Design review of the part built by this model. Coordinates are the model's own, in mm. A direction names the side the tool comes from. Give positions to 0.01 mm unless a question says otherwise; leave off trailing zeros. Write each loop counter-clockwise with the first axis right and the second up, starting at its lowest first coordinate (ties: lowest second). Pieces come first, ordered by that corner, then holes. Notation, with made-up numbers: (21.25, -34) -> (38.25, -34) arc R34 ccw to (38.25, 1) -> close; hole circle Ø10 at (55.25, -35). An arc over 180 degrees is marked (long way). Answer as a JSON object with one key per item and string values.
Autodesk Fusion 360 part; units mm, degrees
sketch "Sketch1" plane through (0, 0, 0) normal (0, 0, 1) x (1, 0, 0)
sketch "Sketch2" plane through (0, 0, 0) normal (0, 0, 1) x (1, 0, 0)
  line L0 (0, 0) -> (24, 0)
  line L1 (24, 0) -> (24, 5)
  line L2 (24, 5) -> (0, 5)
  line L3 (0, 5) -> (0, 0)
  dimension "d157" = 24
  dimension "d158" = 5
extrude "Extrude1" add sketch "Sketch2" along normal blind 70
sketch "Sketch3" plane through (0, 0, 0) normal (0, -1, 0) x (1, 0, 0)
  circle A0 centre (12, 8) radius 3
  line L0 (0, 0) -> (24, 0)
  line L1 (0, 0) -> (0, 70)
  dimension "d161" = 6
  dimension "d162" = 8
  dimension "d163" = 12
extrude "Extrude2" cut sketch "Sketch3" against normal blind 5
sketch "Sketch4" plane through (0, 0, 0) normal (0, -1, 0) x (1, 0, 0)
sketch "Sketch5" plane through (0, 0, 0) normal (0, -1, 0) x (1, 0, 0)
  circle A0 centre (12, 8) radius 3
  dimension "d166" = 6
sketch "Sketch6" plane through (0, 0, 70) normal (0, 0, 1) x (-1, 0, 0)
  line L0 (39, -9) -> (-63, -9)
  line L1 (-63, -9) -> (-63, 37)
  line L2 (-63, 37) -> (39, 37)
  line L3 (39, 37) -> (39, -9)
  line L4 (-24, 0) -> (-24, -5)
  line L5 (-24, -5) -> (0, -5)
  line L6 (33, 4) -> (-57, 4)
  line L7 (-57, 4) -> (-57, 24)
  line L8 (-57, 24) -> (33, 24)
  line L9 (33, 24) -> (33, 4)
  line L10 (0, 0) -> (-24, 0)
  line L11 (39, 32) -> (-63, 32)
  dimension "d167" = 102
  dimension "d168" = 46
  dimension "d169" = 39
  dimension "d170" = 4
  dimension "d171" = 90
  dimension "d172" = 20
  dimension "d173" = 4
  dimension "d174" = 6
  dimension "d175" = 5
extrude "Extrude3" add sketch "Sketch6" along normal blind 5 contours L0 L1 L3 L11
extrude "Extrude4" add sketch "Sketch6" along normal blind 32 contours L1 L2 L3 L11
fillet "Fillet1" radius 2 1 edges at (12, -32, 75)
fillet "Fillet2" radius 1 14 edges at (12, -37, 102) (12, -32, 102) (63, -34.5, 102) (-39, -34.5, 102) (-39, -10.5, 75) (-39, -31.4142, 75.5858) (-39, -32, 89.5) (12, -37, 70) (63, -14, 70) (12, 9, 70) (12, 9, 75) (63, -32, 89.5) (63, -31.4142, 75.5858) (63, -10.5, 75)
sketch "Sketch7" plane through (0, -32, 0) normal (0, 1, 0) x (-1, 0, 0)
  circle A0 centre (-12, 89.7801) radius 3.675
  line L0 (39, 77) -> (39, 101)
  dimension "d184" = 7.35
  dimension "d185" = 51
extrude "Extrude5" cut sketch "Sketch7" against normal blind 5
equation "d163 = d157 / 2"
(1) We need section D-D, the plane y = -2. State the section outline as (x, z) points.
Here are the results:
{"outline": "(-39, 70) -> (62, 70) arc R1 ccw to (63, 71) -> (63, 74) arc R1 ccw to (62, 75) -> (-38, 75) arc R1 ccw to (-39, 74) -> close"}
(2) We need section A-A, the plane x = 12. State the section outline as (y, z) points.
Here are the results:
{"outline": "(-37, 71) arc R1 ccw to (-36, 70) -> (-24, 70) -> (-24, 75) -> (-30, 75) arc R2 cw to (-32, 77) -> (-32, 86.11) -> (-37, 86.11) -> close; (-37, 93.46) -> (-32, 93.46) -> (-32, 101) arc R1 ccw to (-33, 102) -> (-36, 102) arc R1 ccw to (-37, 101) -> close; (-4, 70) -> (0, 70) -> (0, 11) -> (5, 11) -> (5, 70) -> (8, 70) arc R1 ccw to (9, 71) -> (9, 74) arc R1 ccw to (8, 75) -> (-4, 75) -> close; (0, 0) -> (5, 0) -> (5, 5) -> (0, 5) -> close"}
(3) For line 1 along Z through (x, y) = (12, 2.1); line 2 along X through (y, z) = (1.5, 40.5); line 3 along Z through (x, y) = (12, -34), list the stretches that pass through material, from the lowest coordinate up.
Here are the results:
{"line 1": "z = 0 to 5, 11 to 75", "line 2": "x = 0 to 24", "line 3": "z = 70 to 86.11, 93.46 to 102"}
(4) For faces 5 (the flat face through (12, 5, 35)), 6 (the flat face through (12, 0, 35)), 7 (the flat face through (11, -4, 72)), 8 (the flat face through (13, -3, 75)), 9 (the flat face through (24, 2, 35)), list the 3-axis set-ups (+Z, -Z, +X, -X, +Y, -Y) from which the entire face can be reached by the end or side of a thin tool; tool diameter is ignored.
Here are the results:
{"face 5": "-Z, +X, -X, +Y", "face 6": "-Z, +X, -X, -Y", "face 7": "+Z, -Z", "face 8": "+Z, +X, -X, +Y", "face 9": "-Z, +X, +Y, -Y"}
(5) We need section B-B, the plane z = 8. State the section outline as (x, y) points, then the cut area to 3 significant figures.
Here are the results:
{"outline": "(0, 0) -> (9, 0) -> (9, 5) -> (0, 5) -> close; (15, 0) -> (24, 0) -> (24, 5) -> (15, 5) -> close", "area": "90.0 mm²"}
(6) We need section C-C, the plane x = 28. State the section outline as (y, z) points.
Here are the results:
{"outline": "(-37, 71) arc R1 ccw to (-36, 70) -> (-24, 70) -> (-24, 75) -> (-30, 75) arc R2 cw to (-32, 77) -> (-32, 101) arc R1 ccw to (-33, 102) -> (-36, 102) arc R1 ccw to (-37, 101) -> close; (-4, 70) -> (8, 70) arc R1 ccw to (9, 71) -> (9, 74) arc R1 ccw to (8, 75) -> (-4, 75) -> close"}
(7) The part is to be moulded in two halves that separate along X. For faces 1 (the flat face through (13, -24, 72)), 2 (the flat face through (-33, -14, 72)), 3 (the flat face through (13, -37, 86)), 4 (the flat face through (63, -24.1, 73.7)), say which applies: +X half, -X half, draft (parallel to the pull), parting line (faces both ways), or undercut.
Here are the results:
{"face 1": "undercut", "face 2": "undercut", "face 3": "draft", "face 4": "+X half"}
(8) Clearance check with flat-ended pins moving along their axes: pin 1 (8 mm diameter, centred on x = 28, y = -24.5, fed in from -Z); pin 2 (1.5 mm diameter, centred on x = 5, z = 29.5, fed in from -Y); pin 3 (8 mm diameter, centred on x = 25.5, z = 22.5, fed in from +Y); pin 4 (9.5 mm diameter, centred on x = 12, z = 89.78, fed in from -Y). State where each tip first meets the part, or that it passes through.
Here are the results:
{"pin 1": "stops at z = 70", "pin 2": "stops at y = 0", "pin 3": "stops at y = 5", "pin 4": "stops at y = -37"}
